```python
from build123d import *

# Parameters (mm, degrees)
F1_DEPTH = 6
F2_W     = 40
F2_H     = 20
F3_DEPTH = 50
F5_DEPTH = 40
F7_DEPTH = 30
F8_DEPTH = 30


# Not quite as in the source:
# - ends of sketch curves that miss each other by under 0.0002 mm in the source are joined


with BuildPart() as f1:
    # F0 (on Top) → F1 (new body)
    with BuildSketch(Plane.XY):
        with BuildLine():
            ThreePointArc((28.9254424359, -34.4719999404), (40.7838504166, -19.0178217783), (45, 0))
            ThreePointArc((45, 0), (40.7838504166, 19.0178217783), (28.9254424359, 34.4719999404))
            Line((28.9254424359, 34.4719999404), (24.4259291681, 29.1096888385))
            ThreePointArc((24.4259292345, 29.1096887828), (34.4396959257, 16.0594939069), (38, 0))
            ThreePointArc((38, 0), (34.4396959, -16.059493962), (24.4259291412, -29.1096888611))
            Line((24.4259291681, -29.1096888385), (28.9254424359, -34.4719999404))
        make_face()
        with BuildLine():
            ThreePointArc((22.5, -38.9711431703), (25.8109396358, -36.861841993), (28.9254424359, -34.4719999404))
            Line((28.9254424359, -34.4719999404), (24.4259291681, -29.1096888385))
            ThreePointArc((24.4259291412, -29.1096888611), (21.795904567, -31.127777693), (19, -32.9089653438))
            Line((19, -32.9089653438), (22.5, -38.9711431703))
        make_face()
        with BuildLine():
            ThreePointArc((15.3909064497, -42.2861679354), (19.0178217783, -40.7838504166), (22.5, -38.9711431703))
            Line((22.5, -38.9711431703), (19, -32.9089653438))
            ThreePointArc((19, -32.9089653438), (16.0594939837, -34.4396958899), (12.9967655243, -35.7083195615))
            Line((12.9967654464, -35.7083195899), (15.3909064497, -42.2861679354))
        make_face()
        with BuildLine():
            ThreePointArc((-44.3163488855, -7.814167995), (-22.5, -38.9711431703), (15.3909064497, -42.2861679354))
            Line((15.3909064497, -42.2861679354), (12.9967654464, -35.7083195899))
            ThreePointArc((12.9967655243, -35.7083195615), (-18.9999999457, -32.9089653752), (-37.4226946071, -6.5986307931))
            Line((-37.4226946145, -6.5986307513), (-44.3163488855, -7.814167995))
        make_face()
        with BuildLine():
            ThreePointArc((-37.4226946071, -6.5986307931), (-18.9999999457, -32.9089653752), (12.9967655243, -35.7083195615))
            ThreePointArc((12.9967655243, -35.7083195615), (10.6448654939, -35.5803659462), (9.1102432746, -33.7935418013))
            ThreePointArc((9.1102432746, -33.7935418013), (-17.5, -30.3108891325), (-33.8211873211, -9.0070687902))
            ThreePointArc((-33.8211873211, -9.0070687902), (-36.1359334802, -8.5714590704), (-37.4226946071, -6.5986307931))
        make_face()
        with BuildLine():
            ThreePointArc((-33.8211873211, -9.0070687902), (-17.5, -30.3108891325), (9.1102432746, -33.7935418013))
            ThreePointArc((9.1102432746, -33.7935418013), (9.2795808611, -31.5634020763), (10.9446447781, -30.0701637954))
            ThreePointArc((10.9446447781, -30.0701637954), (-15.9999999119, -27.712812972), (-31.5138480965, -5.5567416849))
            ThreePointArc((-31.5138480965, -5.5567416849), (-31.4796872612, -5.8162189899), (-31.4682713554, -6.0776862183))
            ThreePointArc((-31.4682713554, -6.0776862183), (-32.1293344064, -7.956349027), (-33.8211873211, -9.0070687902))
        make_face()
        with BuildLine():
            Line((10.9446445864, -30.0701638651), (0, 0))
            Line((0, 0), (-31.5138480964, -5.5567416853))
            ThreePointArc((-31.5138480964, -5.5567416853), (-15.9999999119, -27.712812972), (10.9446445864, -30.0701638651))
        make_face()
        with BuildLine():
            Line((-31.5138480964, -5.5567416853), (0, 0))
            Line((0, 0), (-32, 0))
            ThreePointArc((-32, 0), (-31.878230339, -2.7889837677), (-31.5138480965, -5.5567416849))
        make_face()
        with BuildLine():
            Line((-32, 0), (0, 0))
            Line((0, 0), (-31.5138480964, 5.5567416853))
            ThreePointArc((-31.5138480966, 5.5567416843), (-31.878230339, 2.7889837674), (-32, 0))
        make_face()
        with BuildLine():
            ThreePointArc((-45, 0), (-44.8287614141, -3.9220084236), (-44.3163488855, -7.814167995))
            Line((-44.3163488855, -7.814167995), (-37.4226946145, -6.5986307513))
            ThreePointArc((-37.4226946071, -6.5986307931), (-37.8553985256, -3.3119182456), (-38, 0))
            Line((-38, 0), (-45, 0))
        make_face()
        with BuildLine():
            Line((-37.4226946145, 6.5986307513), (-44.3163488855, 7.814167995))
            ThreePointArc((-44.3163488855, 7.814167995), (-44.8287614141, 3.9220084236), (-45, 0))
            Line((-45, 0), (-38, 0))
            ThreePointArc((-38, 0), (-37.8553985261, 3.3119182405), (-37.4226946089, 6.5986307831))
        make_face()
        with BuildLine():
            Line((12.9967654464, 35.7083195899), (15.3909064497, 42.2861679354))
            ThreePointArc((15.3909064497, 42.2861679354), (-22.5, 38.9711431703), (-44.3163488855, 7.814167995))
            Line((-44.3163488855, 7.814167995), (-37.4226946145, 6.5986307513))
            ThreePointArc((-37.4226946089, 6.5986307831), (-18.9999999501, 32.9089653726), (12.9967655243, 35.7083195615))
        make_face()
        with BuildLine():
            ThreePointArc((9.1102432746, 33.7935418013), (10.6448654939, 35.5803659462), (12.9967655243, 35.7083195615))
            ThreePointArc((12.9967655243, 35.7083195615), (-18.9999999501, 32.9089653726), (-37.4226946089, 6.5986307831))
            ThreePointArc((-37.4226946089, 6.5986307831), (-36.1359334844, 8.5714590676), (-33.8211873211, 9.0070687902))
            ThreePointArc((-33.8211873211, 9.0070687902), (-17.5, 30.3108891325), (9.1102432746, 33.7935418013))
        make_face()
        with BuildLine():
            Line((-31.5138480964, 5.5567416853), (0, 0))
            Line((0, 0), (10.9446445864, 30.0701638651))
            ThreePointArc((10.9446445864, 30.0701638651), (-15.9999999047, 27.7128129761), (-31.5138480964, 5.5567416853))
        make_face()
        with BuildLine():
            ThreePointArc((10.9446447943, 30.0701637895), (9.2795808649, 31.5634020686), (9.1102432746, 33.7935418013))
            ThreePointArc((9.1102432746, 33.7935418013), (-17.5, 30.3108891325), (-33.8211873211, 9.0070687902))
            ThreePointArc((-33.8211873211, 9.0070687902), (-32.1293344064, 7.956349027), (-31.4682713554, 6.0776862183))
            ThreePointArc((-31.4682713554, 6.0776862183), (-31.4796872612, 5.8162189895), (-31.5138480966, 5.5567416843))
            ThreePointArc((-31.5138480966, 5.5567416843), (-15.9999999047, 27.7128129761), (10.9446447943, 30.0701637895))
        make_face()
        with BuildLine():
            Line((19, 32.9089653438), (22.5, 38.9711431703))
            ThreePointArc((22.5, 38.9711431703), (19.0178217783, 40.7838504166), (15.3909064497, 42.2861679354))
            Line((15.3909064497, 42.2861679354), (12.9967654464, 35.7083195899))
            ThreePointArc((12.9967655243, 35.7083195615), (16.0594939837, 34.4396958899), (19, 32.9089653438))
        make_face()
        with BuildLine():
            Line((24.4259291681, 29.1096888385), (28.9254424359, 34.4719999404))
            ThreePointArc((28.9254424359, 34.4719999404), (25.8109396358, 36.861841993), (22.5, 38.9711431703))
            Line((22.5, 38.9711431703), (19, 32.9089653438))
            ThreePointArc((19, 32.9089653438), (21.7959046168, 31.1277776581), (24.4259292345, 29.1096887828))
        make_face()
        with BuildLine():
            Line((0, 0), (20.56920351, 24.5134221798))
            ThreePointArc((20.5692034907, 24.5134221959), (18.354445953, 26.2128654244), (16, 27.7128129211))
            Line((16, 27.7128129211), (0, 0))
        make_face()
        with BuildLine():
            Line((0, 0), (16, 27.7128129211))
            ThreePointArc((16, 27.7128129211), (13.523784476, 29.0018491384), (10.9446447943, 30.0701637895))
            Line((10.9446447943, 30.0701637895), (0, 0))
        make_face()
        with BuildLine():
            ThreePointArc((32, 0), (29.0018491799, 13.5237843871), (20.5692034907, 24.5134221959))
            Line((20.56920351, 24.5134221798), (0, 0))
            Line((0, 0), (20.56920351, -24.5134221798))
            ThreePointArc((20.5692034979, -24.5134221899), (29.0018491818, -13.5237843828), (32, 0))
        make_face()
        with BuildLine():
            ThreePointArc((16, -27.7128129211), (18.3544459568, -26.2128654218), (20.5692034979, -24.5134221899))
            Line((20.56920351, -24.5134221798), (0, 0))
            Line((0, 0), (16, -27.7128129211))
        make_face()
        with BuildLine():
            Line((16, -27.7128129211), (0, 0))
            Line((0, 0), (10.9446445864, -30.0701638651))
            ThreePointArc((10.9446445864, -30.0701638651), (13.5237844681, -29.0018491421), (16, -27.7128129211))
        make_face()
        with BuildLine():
            ThreePointArc((35, 0), (32.3255552282, 13.4185870786), (24.7109440465, 24.7864730111))
            ThreePointArc((24.7109440465, 24.7864730111), (22.6949176866, 23.8180538062), (20.5692034907, 24.5134221959))
            ThreePointArc((20.5692034907, 24.5134221959), (29.0018491799, 13.5237843871), (32, 0))
            ThreePointArc((32, 0), (29.0018491818, -13.5237843828), (20.5692034979, -24.5134221899))
            ThreePointArc((20.5692034979, -24.5134221899), (22.6949176913, -23.8180538065), (24.7109440465, -24.7864730111))
            ThreePointArc((24.7109440465, -24.7864730111), (32.3255552282, -13.4185870786), (35, 0))
        make_face()
        with BuildLine():
            ThreePointArc((38, 0), (34.4396959257, 16.0594939069), (24.4259292345, 29.1096887828))
            ThreePointArc((24.4259292345, 29.1096887828), (25.2164897185, 28.0794102551), (25.497566339, 26.8115555092))
            ThreePointArc((25.497566339, 26.8115555092), (25.294004531, 25.7253080978), (24.7109440465, 24.7864730111))
            ThreePointArc((24.7109440465, 24.7864730111), (32.3255552282, 13.4185870786), (35, 0))
            ThreePointArc((35, 0), (32.3255552282, -13.4185870786), (24.7109440465, -24.7864730111))
            ThreePointArc((24.7109440465, -24.7864730111), (25.294004531, -25.7253080978), (25.497566339, -26.8115555092))
            ThreePointArc((25.497566339, -26.8115555092), (25.2164896927, -28.0794103103), (24.4259291412, -29.1096888611))
            ThreePointArc((24.4259291412, -29.1096888611), (34.4396959, -16.059493962), (38, 0))
        make_face()
    extrude(amount=F1_DEPTH)

    # F2 (on face) → F3 (join)
    with BuildSketch(Plane.XY.offset(6)):
        Rectangle(F2_W, F2_H)
    extrude(amount=F3_DEPTH)

    # F4 (on face) → F5 (join)
    with BuildSketch(Plane(origin=(-20, 0, 0), x_dir=(0, -1, 0), z_dir=(-1, 0, 0))):
        Polygon((10, 14), (10, 6), (18, 6), align=None)
        Polygon((-10, 14), (-20, 6), (-10, 6), align=None)
    extrude(amount=-F5_DEPTH)

    # F6 (on face) → F7 (cut)
    with BuildSketch(Plane.XZ.offset(10)):
        with BuildLine():
            Line((-14.1421356237, 50.1421356237), (-20, 56))
            Line((-20, 56), (-20, 36))
            ThreePointArc((-20, 36), (-18.4775906502, 43.6536686473), (-14.1421356237, 50.1421356237))
        make_face()
        with BuildLine():
            Line((1.654e-07, 56), (-20, 56))
            Line((-20, 56), (-14.1421356237, 50.1421356237))
            ThreePointArc((-14.1421356237, 50.1421356237), (-7.6536685709, 54.4775906819), (1.654e-07, 56))
        make_face()
        with BuildLine():
            Line((20, 56), (1.654e-07, 56))
            ThreePointArc((1.654e-07, 56), (7.6536687237, 54.4775906186), (14.1421356237, 50.1421356237))
            Line((14.1421356237, 50.1421356237), (20, 56))
        make_face()
        with BuildLine():
            Line((20, 56), (14.1421356237, 50.1421356237))
            ThreePointArc((14.1421356237, 50.1421356237), (18.4775906502, 43.6536686473), (20, 36))
            Line((20, 36), (20, 56))
        make_face()
    extrude(amount=-F7_DEPTH, mode=Mode.SUBTRACT)

    # F6 (on face) → F8 (cut)
    with BuildSketch(Plane.XZ.offset(10)):
        with BuildLine():
            Line((0, 36), (-3.1819805153, 39.1819805153))
            ThreePointArc((-3.1819805153, 39.1819805153), (-1.7220754456, 31.8425421037), (4.5, 36))
            ThreePointArc((4.5, 36), (4.1574578963, 37.7220754456), (3.1819805153, 39.1819805153))
            Line((3.1819805153, 39.1819805153), (0, 36))
        make_face()
        with BuildLine():
            ThreePointArc((3.1819805153, 39.1819805153), (0, 40.5), (-3.1819805153, 39.1819805153))
            Line((-3.1819805153, 39.1819805153), (0, 36))
            Line((0, 36), (3.1819805153, 39.1819805153))
        make_face()
    extrude(amount=-F8_DEPTH, mode=Mode.SUBTRACT)


solid = f1.part
```
Source: CAD feature listing. Evaluate the final solid. Frame: model axes, mm. A direction names the side the tool comes from. Give positions to 0.01 mm unless a question says otherwise; leave off trailing zeros. Loops run counter-clockwise (first coordinate to the right, second up) from the corner with the lowest first, then second, coordinate; pieces in that order, holes last. Notation, with made-up numbers: (77, 30.25) -> (100, 30.25) arc R23 ccw to (100, 62.25) -> close; hole circle Ø7 at (12, 9). An arc over 180 degrees is marked (long way). Use a Markdown table: item, result. Add a question column.
(1) Section query B-B (x = -8.5). Output: boundary loops of the cut face in (y, z).
(2) First-contact query: pin 1 Ø8 at (x, y) = (-26, -9.5) entering from +Z; pin 2 Ø15 at (y, z) = (-4, 20) entering from -X; pin 3 Ø24 at (y, z) = (6.5, 26.5) entering from +X. Flat tips, straight axial feed; report the tip coordinate or a pass-through.
(3) Section query D-D (y = -15). Output: boundary loops of the cut face in (x, z), then the cut area to 3 significant figures.
(4) Access query for faces 1 (the face through (0, 10, 30)), 2 (the face through (-1, 1, 0)). Directions: +Z, -Z, +X, -X, +Y, -Y. A direction counts if a zero-diameter tool reaches every point of the face in a straight line with its end or side. Return the directions, or none.
(5) Pull-direction query (X, two-part tool) for faces 3 (the face through (0, -10, 30)), 4 (the face through (16.07, 27.67, 2.96)), 5 (the face through (-20, 1, 21)), 6 (the face through (20, 1, 21)); classes: +X half, -X half, draft (parallel to the pull), parting line (faces both ways), or undercut.
(6) Section query C-C (z = 9). Output: boundary loops of the cut face in (x, y).
(7) Ray query, line 1 (X direction, y = -5.25, z = 36); line 2 (Z direction, x = 24, y = 2); line 3 (Y direction, x = -0.5, z = 20). Return the intervals inside material, ascending.
(8) Section query A-A (y = -3). Output: boundary loops of the cut face in (x, z).
Checked values:
| question | item | result |
|---|---|---|
| 1 | outline | (-44.19, 0) -> (44.19, 0) -> (44.19, 6) -> (20, 6) -> (10, 14) -> (10, 54.1) -> (-10, 54.1) -> (-10, 14) -> (-18, 6) -> (-44.19, 6) -> close |
| 2 | pin 1 | z = 6 |
| 2 | pin 2 | x = -20 |
| 2 | pin 3 | x = 20 |
| 3 | outline | (-42.43, 0) -> (42.43, 0) -> (42.43, 6) -> (20, 6) -> (20, 9) -> (-20, 9) -> (-20, 6) -> (-42.43, 6) -> close |
| 3 | area | 629 mm^2 |
| 4 | face 1 | +Z, +X, -X, +Y |
| 4 | face 2 | -Z, +X, -X, +Y, -Y |
| 5 | face 3 | draft |
| 5 | face 4 | undercut |
| 5 | face 5 | -X half |
| 5 | face 6 | +X half |
| 6 | outline | (-20, -15) -> (20, -15) -> (20, 16.25) -> (-20, 16.25) -> close |
| 7 | line 1 | -20 to -4.5, 4.5 to 20 |
| 7 | line 2 | 0 to 6 |
| 7 | line 3 | -10 to 10 |
| 8 | outline | (-44.9, 0) -> (-37.88, 0) -> (-37.88, 6) -> (-44.9, 6) -> close; (-31.86, 0) -> (44.9, 0) -> (44.9, 6) -> (20, 6) -> (20, 36) arc R20 ccw to (-20, 36) -> (-20, 6) -> (-31.86, 6) -> close; hole circle Ø9 at (0, 36) |
